Can you work these out from the model? Positions are in its coordinate system, mm. Coordinates: 2 decimals unless noted, no trailing zeros. Order: outer loops, then holes, each group sorted by start corner. A loop starts at its lowest first (then second) coordinate and runs counter-clockwise, first axis right, second up.
```python
from build123d import *

# Parameters (mm, degrees)
BOSS_EXTRUDE1_DEPTH = 2
BOSS_EXTRUDE2_DEPTH = 2


with BuildPart() as part:
    # Sketch1 → Boss-Extrude1 (new body)
    with BuildSketch(Plane(origin=(0, 0, 0), x_dir=(0, 0, -1), z_dir=(1, 0, 0))):
        Polygon((-7.5, 3.15), (-7.5, 5.15), (-2.5, 5.15), (-2.5, 3.15), (2.5, 3.15), (2.5, 5.15), (7.5, 5.15), (7.5, 3.15), (10, 3.15), (10, -3.15), (7.5, -3.15), (7.5, -5.15), (2.5, -5.15), (2.5, -3.15), (-2.5, -3.15), (-2.5, -5.15), (-7.5, -5.15), (-7.5, -3.15), (-10, -3.15), (-10, 3.15), align=None)
    extrude(amount=BOSS_EXTRUDE1_DEPTH)

    # Sketch2 → Boss-Extrude2 (add)
    with BuildSketch(Plane(origin=(2, 0, 0), x_dir=(0, 0, -1), z_dir=(1, 0, 0))):
        Polygon((-10, -5.15), (10, -5.15), (10, -35.15), (7.5, -35.15), (7.5, -33.15), (2.5, -33.15), (2.5, -35.15), (-2.5, -35.15), (-2.5, -33.15), (-7.5, -33.15), (-7.5, -35.15), (-10, -35.15), align=None)
    extrude(amount=-BOSS_EXTRUDE2_DEPTH)


solid = part.part
```
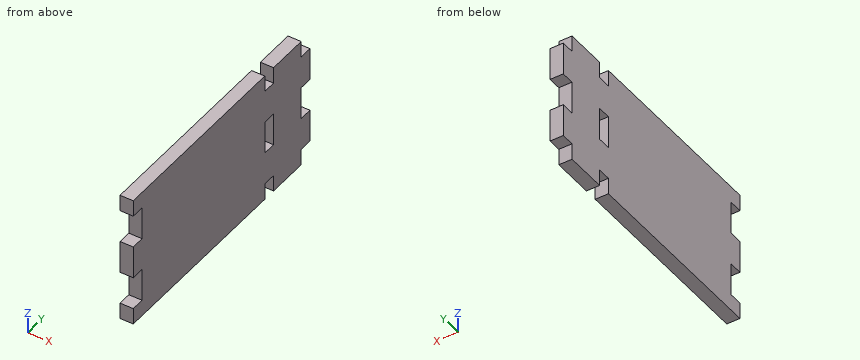
1. Imagine slicing it at A-A on z = 8.5. Please give me the cut outline in (x, y).
Completed:
outline: (0, -35.15) - (2, -35.15) - (2, -5.15) - (0, -5.15) - close; (0, -3.15) - (2, -3.15) - (2, 3.15) - (0, 3.15) - close
2. I'm going to push flat-ended pins straight in: pin 1 (1 mm diameter, centred on x = 1, y = -4, fed in from -Z); pin 2 (0.6 mm diameter, centred on x = 1.5, y = -4.5, fed in from +Z); pin 3 (1 mm diameter, centred on x = 1, z = -0.5, fed in from +Y). Where does each tip first touch, or does it pass through?
Completed:
pin 1: stops at z = -7.5
pin 2: stops at z = 7.5
pin 3: stops at y = 3.15
3. Imagine slicing it at C-C on z = 4.75. Please give me the cut outline in (x, y), then the cut area to 3 significant figures.
Completed:
outline: (0, -33.15) - (2, -33.15) - (2, 5.15) - (0, 5.15) - close
area: 76.6 mm2
4. Please list where these lines run through material, in increasing order: probe 1 along Y at (x, z) = (0.35, -8.5); probe 2 along Y at (x, z) = (0.8, 6).
Completed:
probe 1: y = -35.15 to -5.15, -3.15 to 3.15
probe 2: y = -33.15 to 5.15
